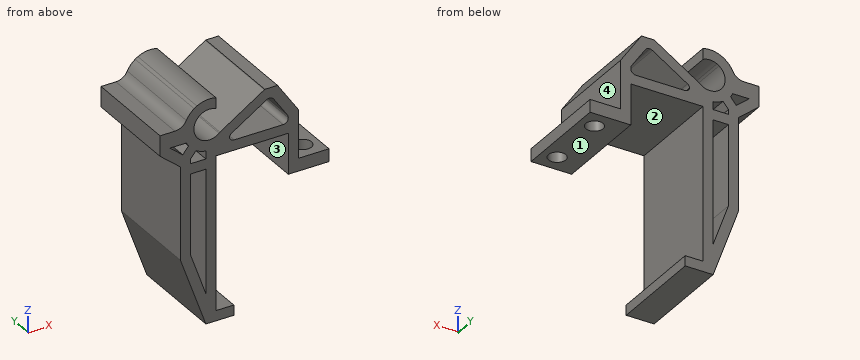
from build123d import *

# Parameters (mm, degrees)
F0_W        = 3
F0_H        = 2
F1_DEPTH    = 19
F3_D        = 3.4
F4_T1_DEPTH = 19


# Not quite as in the source:
# - a fillet or chamfer that OpenCascade refuses, or shapes differently, is made with other operations: its cross-section is extruded or revolved along the edge and cut away or added


with BuildPart() as f1:
    # F0 (on Front) → F1 (new body)
    with BuildSketch(Plane.XZ):
        with Locations((-7, 31.2)):
            Rectangle(F0_W, F0_H)
        with BuildLine():
            Line((-10.0427465571, 34.4155443421), (-8.5, 33.1427784325))
            Line((-8.5, 33.1427784325), (-7.441074238, 34.4263248107))
            ThreePointArc((-7.441074238, 34.4263248107), (-8.244619139, 35.032889635), (-8.9103596286, 35.7881345584))
            Line((-8.9103596286, 35.7881345584), (-10.0427465571, 34.4155443421))
        make_face()
        with BuildLine():
            Line((-10.5, 14), (-5.5, 0))
            Line((-5.5, 0), (-5.5, 5.9464274989))
            Line((-5.5, 5.9464274989), (-8.5, 14.3464274989))
            Line((-8.5, 14.3464274989), (-8.5, 30.2))
            Line((-8.5, 30.2), (-8.5, 32.2))
            Line((-8.5, 32.2), (-8.5, 33.1427784325))
            Line((-8.5, 33.1427784325), (-10.0427465571, 34.4155443421))
            Line((-10.0427465571, 34.4155443421), (-10.7699806475, 35.0155124667))
            Line((-10.7699806475, 35.0155124667), (-12.5, 36.4427784325))
            Line((-12.5, 36.4427784325), (-12.5, 36.5))
            Line((-12.5, 36.5), (-9.3357403136, 36.5))
            ThreePointArc((-9.3357403136, 36.5), (-9.7907115521, 37.9601557031), (-9.7830217401, 39.4895328221))
            ThreePointArc((-9.7830217401, 39.4895328221), (-9.7333018776, 39.7544433664), (-9.6693788597, 40.0162897125))
            ThreePointArc((-9.6693788597, 40.0162897125), (-9.5234750406, 40.4660413374), (-9.3357403136, 40.9))
            ThreePointArc((-9.3357403136, 40.9), (-10.2578590901, 39.8786796564), (-11.5807347457, 39.5))
            Line((-11.5807347457, 39.5), (-14.5, 39.5))
            Line((-14.5, 39.5), (-14.5, 35.5))
            Line((-14.5, 35.5), (-10.5, 32.2))
            Line((-10.5, 32.2), (-10.5, 14))
        make_face()
        with BuildLine():
            Line((-4.3254974298, 0), (0, 0))
            Line((0, 0), (0, 2))
            Line((0, 2), (-3.5, 2))
            Line((-3.5, 2), (-3.5, 32.2))
            Line((-3.5, 32.2), (6, 32.2))
            Line((6, 32.2), (10.7, 32.2))
            Line((10.7, 32.2), (10.7, 24.2))
            Line((10.7, 24.2), (18.7, 24.2))
            Line((18.7, 24.2), (18.7, 26.7))
            Line((18.7, 26.7), (12.7, 26.7))
            Line((12.7, 26.7), (12.7, 36.2))
            Line((12.7, 36.2), (8.5871078054, 42.2))
            Line((8.5871078054, 42.2), (6.0871078054, 42.2))
            Line((6.0871078054, 42.2), (6, 42.14441707))
            Line((6, 42.14441707), (-2.7279451008, 36.5751714729))
            ThreePointArc((-2.7279451008, 36.5751714729), (-2.80839002, 36.4979195279), (-2.8916508552, 36.4237111635))
            ThreePointArc((-2.8916508552, 36.4237111635), (-7.1777694161, 36.8127553939), (-6.6645515402, 41.085784196))
            ThreePointArc((-6.6645515402, 41.085784196), (-6.4594906698, 41.2290009349), (-6.2432123403, 41.3546380278))
            ThreePointArc((-6.2432123403, 41.3546380278), (-4.8748228701, 41.6998591388), (-3.5, 41.3812223027))
            Line((-3.5, 41.3812223027), (-3.5, 43.5154909445))
            ThreePointArc((-3.5, 43.5154909445), (-5.4216118426, 43.6667277767), (-7.2576401277, 43.0798165491))
            Line((-7.2576401277, 43.0798165491), (-7.8017760466, 42.7326069212))
            ThreePointArc((-7.8017760466, 42.7326069212), (-8.6798603613, 41.909300368), (-9.3357403136, 40.9))
            ThreePointArc((-9.3357403136, 40.9), (-9.5234750406, 40.4660413374), (-9.6693788597, 40.0162897125))
            ThreePointArc((-9.6693788597, 40.0162897125), (-9.7333018776, 39.7544433664), (-9.7830217401, 39.4895328221))
            ThreePointArc((-9.7830217401, 39.4895328221), (-9.7907115521, 37.9601557031), (-9.3357403136, 36.5))
            ThreePointArc((-9.3357403136, 36.5), (-9.1378337815, 36.1352330993), (-8.9103596286, 35.7881345584))
            ThreePointArc((-8.9103596286, 35.7881345584), (-8.244619139, 35.032889635), (-7.441074238, 34.4263248107))
            ThreePointArc((-7.441074238, 34.4263248107), (-6.506072339, 33.9837160238), (-5.5, 33.7429889213))
            Line((-5.5, 33.7429889213), (-5.5, 32.3898009956))
            Line((-5.5, 32.3898009956), (-5.5, 32.2))
            Line((-5.5, 32.2), (-5.5, 30.2))
            Line((-5.5, 30.2), (-5.5, 5.9464274989))
            Line((-5.5, 5.9464274989), (-5.5, 0))
            Line((-5.5, 0), (-4.3254974298, 0))
        make_face()
        Polygon((-0.9128921946, 34.2), (-0.9128921946, 35.3608666872), (6.6708440859, 40.2), (7.5332950832, 40.2), (10.7, 35.5803239662), (10.7, 34.2), align=None, mode=Mode.SUBTRACT)
    extrude(amount=F1_DEPTH)

    # F3 (through all)
    with Locations(Plane.XY.offset(26.7)):
        with Locations((15.7, -15.5), (15.7, -3.5)):
            Hole(F3_D / 2)

    # F4: fillet of radius 1 on 6 edges, made by hand

    # F4_s2 → F4_t1 (join)
    with BuildSketch(Plane.XZ):
        with BuildLine():
            ThreePointArc((10.5248181897, 35.8358839984), (10.6552010756, 35.5664435563), (10.7, 35.2704859494))
            Line((10.7, 35.2704859494), (10.7, 35.5803239662))
            Line((10.7, 35.5803239662), (10.5248181897, 35.8358839984))
        make_face()
        with BuildLine():
            ThreePointArc((7.0063887221, 40.2), (7.4725442492, 40.0847027888), (7.8312069118, 39.7653980491))
            Line((7.8312069118, 39.7653980491), (7.5332950832, 40.2))
            Line((7.5332950832, 40.2), (7.0063887221, 40.2))
        make_face()
        with BuildLine():
            ThreePointArc((6.4247991527, 40.0430003116), (6.6825339897, 40.1599479964), (6.9627122262, 40.2))
            Line((6.9627122262, 40.2), (6.6708440859, 40.2))
            Line((6.6708440859, 40.2), (6.4247991527, 40.0430003116))
        make_face()
        with BuildLine():
            ThreePointArc((-0.9128921946, 34.8127210695), (-0.7897938633, 35.2933908764), (-0.450805268, 35.6557213811))
            Line((-0.450805268, 35.6557213811), (-0.9128921946, 35.3608666872))
            Line((-0.9128921946, 35.3608666872), (-0.9128921946, 34.8127210695))
        make_face()
        with BuildLine():
            ThreePointArc((0.0871078054, 34.2), (-0.6199989757, 34.4928932188), (-0.9128921946, 35.2))
            Line((-0.9128921946, 35.2), (-0.9128921946, 34.2))
            Line((-0.9128921946, 34.2), (0.0871078054, 34.2))
        make_face()
        with BuildLine():
            ThreePointArc((9.7, 34.2), (10.4071067812, 34.4928932188), (10.7, 35.2))
            Line((10.7, 35.2), (10.7, 34.2))
            Line((10.7, 34.2), (9.7, 34.2))
        make_face()
    extrude(amount=F4_T1_DEPTH)


solid = f1.part
For this review, take the finished solid that the model builds, in its own axes (mm). Face numbers are marked on the shaded views. A direction names the side the tool comes from. Round coordinates to 2 decimals unless told otherwise and drop trailing zeros. Write each loop counter-clockwise with the first axis right and the second up, starting at its lowest first coordinate (ties: lowest second). Pieces come first, ordered by that corner, then holes. Notation, with made-up numbers: (81.5, 79) - (111.5, 79) arc R11 cw to (111.5, 89) - close; hole circle Ø1 at (71.25, 33). An arc over 180 degrees is marked (long way). Write item = value, one per line. Start each with the question number.
1. Wall thickness on L1, parallel to Y at x = 15.7, z = 25; L2, parallel to X at y = -9.25, z = 24.5; L3, parallel to Y at x = 15, z = 25: over which ranges is each line inside the solid? List them lowest first.
2. Consider section D-D on z = 38.7. State the section outline as (x, y) points.
3. Consider section A-A on x = 15.7. State the section outline as (y, z) points, plus the area to 3 significant figures.
4. Consider section C-C on y = -15.5. Give the number of separate pieces and of enclosed holes in the cut face, plus the area to 3 significant figures.
5. For pin 1 Ø0.9 at (x, y) = (-12.5, -10.5) entering from +Z; pin 2 Ø4 at (x, y) = (13.5, -13.5) entering from +Z; pin 3 Ø5 at (x, y) = (3, -14) entering from +Z, all flat-tipped, find the tip position at first contact; note any pin that passes through.
6. Consider section B-B on z = 31. State the section outline as (x, y) points, plus the area to 3 significant figures.
7. For the marked faces 1, 2, 3 and 4, list the 3-axis set-ups (+Z, -Z, +X, -X, +Y, -Y) from which the entire face can be reached by the end or side of a thin tool; tool diameter is ignored.
Evaluation:
q1.L1 = -19 to -17.2, -13.8 to -5.2, -1.8 to 0
q1.L2 = -10.5 to -8.5, -5.5 to -3.5, 10.7 to 18.7
q1.L3 = -19 to -17.05, -13.95 to -5.05, -1.95 to 0
q2.outline = (-14.5, -19) - (-7.85, -19) - (-7.85, 0) - (-14.5, 0) - close; (0.6, -19) - (4.32, -19) - (4.32, 0) - (0.6, 0) - close; (8.56, -19) - (10.99, -19) - (10.99, 0) - (8.56, 0) - close
q3.outline = (-19, 24.2) - (-17.2, 24.2) - (-17.2, 26.7) - (-19, 26.7) - close; (-13.8, 24.2) - (-5.2, 24.2) - (-5.2, 26.7) - (-13.8, 26.7) - close; (-1.8, 24.2) - (0, 24.2) - (0, 26.7) - (-1.8, 26.7) - close
q3.area = 30.5 mm2
q4.separate_pieces = 2
q4.enclosed_holes = 4
q4.area = 301 mm2
q5.pin_1 = 39.5
q5.pin_2 = 37.95
q5.pin_3 = 41.83
q6.outline = (-10.5, -19) - (-3.5, -19) - (-3.5, 0) - (-10.5, 0) - close; (10.7, -19) - (12.7, -19) - (12.7, 0) - (10.7, 0) - close
q6.area = 171 mm2
q7.face_1 = -Z, +X, +Y, -Y
q7.face_2 = +Y, -Y
q7.face_3 = -Z, +Y, -Y
q7.face_4 = +Z, +X, +Y, -Y
